Read the model definition and answer for the solid it produces. Units are mm, in the model's axes. A direction names the side the tool comes from. Give positions to 0.01 mm unless a question says otherwise; leave off trailing zeros.
Item 1: Which of the six approach directions +Z, -Z, +X, -X, +Y, -Y give full straight-line access (tool end or side, diameter ignored) to faces 1 (the face through (-98, 1, 1.689)), 2 (the face through (-23, 1, 0))?
Item 2: Find the intervals of material crossed by line 1 along Z through (x, y) = (-76, 57); line 2 along X through (y, z) = (-37.5, 0.5); line 3 along Z through (x, y) = (95.5, 0), in increasing order.
Item 3: Given pin 1 Ø8 at (x, y) = (-64.5, -49.5) entering from -Z; pin 2 Ø0.9 at (x, y) = (51.5, -20) entering from -Z; pin 3 Ø1.9 at (x, z) = (-76.2, 3.175) entering from -Y; pin 4 Ø1.9 at (y, z) = (0, 3.175) entering from +X, each flat-ended and moving along its own axis, determine where each tip first touches the part or whether it passes through.
Autodesk Inventor part; units mm, degrees
ref_plane "YZ Plane" through (0, 0, 0) normal (1, 0, 0) x (0, 1, 0)
ref_plane "XZ Plane" through (0, 0, 0) normal (0, 1, 0) x (-1, 0, 0)
ref_plane "XY Plane" through (0, 0, 0) normal (0, 0, 1) x (1, 0, 0)
sketch "Sketch1" plane through (0, 0, 0) normal (0, 0, 1) x (1, 0, 0)
  line L0 (-101.6, -63.5) -> (101.6, -63.5)
  line L1 (101.6, -63.5) -> (101.6, 63.5)
  line L2 (101.6, 63.5) -> (-101.6, 63.5)
  line L3 (-101.6, 63.5) -> (-101.6, -63.5)
  line L4 (-101.6, -63.5) -> (101.6, 63.5) construction
  line L5 (101.6, -63.5) -> (-101.6, 63.5) construction
  point P0 (0, 0)
  dimension "d0" = 203.2
  dimension "d1" = 127
extrude "Extrusion1" add sketch "Sketch1" along normal blind 6.35
sketch "Sketch16" plane through (0, 0, 0) normal (0, 0, -1) x (-1, 0, 0)
  line L0 (-101.6, 63.5) -> (101.6, 63.5)
  line L1 (101.6, -63.5) -> (-101.6, -63.5)
  line L2 (-52.578, 63.5) -> (-50.8, 63.5)
  line L3 (-50.8, 63.5) -> (-50.8, -63.5)
  line L4 (-50.8, -63.5) -> (-52.578, -63.5)
  line L5 (-52.578, -63.5) -> (-52.578, 63.5)
  line L6 (-101.6, -63.5) -> (-101.6, 63.5)
  point P0 (0, 0)
  dimension "d114" = 1.778
  dimension "d115" = 49.022
extrude "Extrusion9" cut sketch "Sketch16" against normal blind 1.6891 contours L0 L3 L1 L5
sketch "Sketch17" plane through (-101.6, 63.5, 6.35) normal (0, 1, 0) x (1, 0, 0)
  line L0 (154.178, 6.35) -> (154.178, 4.6609)
  line L1 (154.178, 4.6609) -> (152.4, 4.6609)
  line L2 (152.4, 4.6609) -> (152.4, 6.35)
  line L3 (152.4, 6.35) -> (0, 6.35)
  line L4 (0, 6.35) -> (0, 0)
  line L5 (203.2, 0) -> (0, 0)
  line L6 (203.2, 6.35) -> (203.2, 0)
  line L7 (203.2, 6.35) -> (154.178, 6.35)
  point P0 (101.6, 6.35)
  point P1 (177.8, 3.175)
  point P2 (25.4, 3.175)
  dimension "d118" = 25.4
  dimension "d119" = 25.4
  dimension "d120" = 3.175
  dimension "d121" = 3.175
hole "Hole7" at (76.2, 63.5, 3.175) at (-76.2, 63.5, 3.175) direction (0, -1, 0) diameter 2.159 depth 8.8646 tip angle 118
mirror "Mirror5" about plane through (0, 0, 0) normal (0, 1, 0) of "Hole7"
sketch "Sketch18" plane through (0, 0, 0) normal (0, 0, -1) x (-1, 0, 0)
  line L0 (-50.8, 63.5) -> (-50.8, -63.5)
  line L1 (101.6, -63.5) -> (-50.8, -63.5)
  line L2 (101.6, 63.5) -> (101.6, -63.5)
  line L3 (-50.8, 63.5) -> (101.6, 63.5)
  line L4 (-101.6, 63.5) -> (101.6, 63.5)
  line L5 (95.1992, 63.5) -> (101.6508, 63.5)
  line L6 (101.6508, 63.5) -> (101.6508, -63.5)
  line L7 (101.6508, -63.5) -> (95.1992, -63.5)
  line L8 (95.1992, -63.5) -> (95.1992, 63.5)
  point P0 (0, 0)
  dimension "d129" = 6.4516
  dimension "d130" = 152.4508
extrude "Extrusion10" cut sketch "Sketch18" against normal blind 1.6891 contours L3 L2 L1 L8 | L5 L6 L7 L2
sketch "Sketch19" plane through (101.6, -63.5, 0) normal (1, 0, 0) x (0, 0, -1)
  line L0 (0, 0) -> (0, 127)
  line L1 (0, 127) -> (-6.35, 127)
  line L2 (-6.35, 0) -> (-6.35, 127)
  line L3 (0, 0) -> (-6.35, 0)
  point P0 (0, 63.5)
  point P1 (-3.175, 63.5)
  dimension "d133" = 3.175
  dimension "d134" = 63.5
hole "Hole8" at (101.6, 0, 3.175) direction (-1, 0, 0) diameter 2.159 depth 8.8646 tip angle 118
equation "\"width\" = 127"
equation "\"depth\" = 203.2"
equation "\"aerogelHolderDepth\" = 49.022"
equation "\"caseThickness\" = 6.35"
equation "\"alignmentGrooveDepth\" = 1.5875"
equation "\"height\" = 127"
equation "\"mirrorAngle\" = 2.5deg"
equation "\"mirrorThickness\" = 3.175"
equation "\"fresnelThickness\" = 0.254"
equation "\"focalLength\" = 152.4"
equation "\"ior\" = 1.49"
equation "\"centerThickness\" = 1.27"
equation "\"fresnelAngle\" = 90deg"
equation "\"fresnelEffectiveDiameter\" = 152.4"
equation "\"alignmentGrooveClearance\" = 0.1016"
equation "\"frontPanelThickness\" = 1.5875"
equation "\"fresnelGrooveWidth\" = 1.778"
properties part number "topBottom" material "Aluminum 6061"
Response values:
1. face 1: -Z, -X, +Y, -Y
1. face 2: -Z, +X, -X, +Y, -Y
2. line 1: z = 0 to 2.11, 4.24 to 6.35
2. line 2: x = -95.2 to 50.8, 52.58 to 101.6
2. line 3: z = 0 to 2.1, 4.25 to 6.35
3. pin 1: stops at z = 0
3. pin 2: stops at z = 1.69
3. pin 3: stops at y = -54.56
3. pin 4: stops at x = 92.66
